from build123d import *

# Parameters (mm, degrees)
CYLINDER019_R             = 1.25
CYLINDER019_DEPTH         = 10
EXTRUDE002_DEPTH          = 16
FILLET_R                  = 5
FILLET001_R               = 2
FUSION001_PLACEMENT_ANGLE = 180


with BuildPart() as cylinder019:
    # Cylinder019 → Cylinder019 (new body)
    with BuildSketch(Plane(origin=(18.75, 47.98, 6), x_dir=(1, 0, 0), z_dir=(0, 1, 0))):
        Circle(CYLINDER019_R)
    extrude(amount=CYLINDER019_DEPTH)


with BuildPart() as gps002:
    # Sketch016 → Extrude002 (new body)
    with BuildSketch(Plane.XY):
        Polygon((5.88, 0), (31.63, 0), (37.5, 7.5), (37.5, 48), (0, 48), (0, 7.5), align=None)
    extrude(amount=EXTRUDE002_DEPTH)

    # Fillet
    fillet_edges = [gps002.edges().sort_by_distance(p)[0] for p in [
        (18.755, 0, 16),
        (34.565, 3.75, 16),
        (37.5, 27.75, 16),
        (18.75, 48, 16),
        (0, 27.75, 16),
        (2.94, 3.75, 16),
    ]]
    fillet(fillet_edges, radius=FILLET_R)

    # Fillet001
    fillet001_edges = [gps002.edges().sort_by_distance(p)[0] for p in [
        (5.88, 0, 5.5),
        (31.63, 0, 5.5),
        (0, 7.5, 5.5),
        (37.5, 7.5, 5.5),
        (0, 48, 5.5),
        (37.5, 48, 5.5),
    ]]
    fillet(fillet001_edges, radius=FILLET001_R)

    # Fusion001: union Cylinder019
    add(cylinder019.part)


with BuildPart() as gps002_1:
    # Fusion001 placement: moved
    add(gps002.part.moved(Location((91.67, 220, 40))).rotate(Axis((91.67, 220, 40), (0, 0, 1)), FUSION001_PLACEMENT_ANGLE))


solid = gps002_1.part
Input: part model. Units: mm. Frame: model coordinates. A direction names the side the tool comes from. Give positions to 0.01 mm unless a question says otherwise; leave off trailing zeros. Loops run counter-clockwise (first coordinate to the right, second up) from the corner with the lowest first, then second, coordinate; pieces in that order, holes last. Notation, with made-up numbers: M 6.25,3.5 L 15.25,3.5 A26 ccw 15.25,35.5 Z; hole C 49.5,32 d2. An arc over 180 degrees is marked long. Use CSV: the item, a comma, the result in double quotes.
(1) Material intervals for L1, parallel to Y at x = 73.5, z = 41.5; L2, parallel to Z at x = 58, y = 191.5; L3, parallel to X at y = 197, z = 55, sorted ascending. Write a range as [from, to].
Outcome:
L1,"y = [172, 220]"
L2,"z = [40, 55.86]"
L3,"x = [56.17, 89.67]"
(2) Section C-C, the plane y = 192.5. Return loops of the section in (x, z).
Outcome:
outline,"M 54.17,40 L 91.67,40 L 91.67,51 A5 ccw 86.67,56 L 59.17,56 A5 ccw 54.17,51 Z"
(3) Section A-A, the plane x = 72.92. Return loops of the section in (y, z).
Outcome:
outline,"M 162.02,44.75 L 172,44.75 L 172,40 L 220,40 L 220,51 A5 ccw 215,56 L 177,56 A5 ccw 172,51 L 172,47.25 L 162.02,47.25 Z"
(4) Pin query (flat end, axial travel): P1, Ø1, axis at x = 58.5, z = 53, coming from the +Y side; P2, Ø8, axis at x = 61, z = 44, coming from the -Y side. Return the tip coordinate at first contact, or that it passes through.
Outcome:
P1,"stops at y = 218.07"
P2,"stops at y = 172"
(5) Section B-B, the plane z = 50.25. Return loops of the section in (x, y).
Outcome:
outline,"M 54.17,174 A2 ccw 56.17,172 L 89.67,172 A2 ccw 91.67,174 L 91.67,211.81 A2 ccw 91.24,213.04 L 86.39,219.23 A2 ccw 84.82,220 L 61.01,220 A2 ccw 59.44,219.23 L 54.6,213.04 A2 ccw 54.17,211.81 Z"
(6) Set-up query: faces 1 (the face through (73.08, 167.08, 44.76)), 2 (the face through (55.6, 192.6, 54.5)). Return all of +Z, -Z, +X, -X, +Y, -Y with unobstructed straight access to the full face (end or side cutting, diameter ignored); none if empty.
Outcome:
face 1,"-Y"
face 2,"+Z, -X, +Y, -Y"
(7) Section D-D, the plane z = 46. Return loops of the section in (x, y).
Outcome:
outline,"M 54.17,174 A2 ccw 56.17,172 L 71.67,172 L 71.67,162.02 L 74.17,162.02 L 74.17,172 L 89.67,172 A2 ccw 91.67,174 L 91.67,211.81 A2 ccw 91.24,213.04 L 86.39,219.23 A2 ccw 84.82,220 L 61.01,220 A2 ccw 59.44,219.23 L 54.6,213.04 A2 ccw 54.17,211.81 Z"
